For this review, take the finished solid that the model builds, in its own axes (mm). A direction names the side the tool comes from. Coordinates: 2 decimals unless noted, no trailing zeros. Write each loop counter-clockwise with the first axis right and the second up, starting at its lowest first coordinate (ties: lowest second). Pieces come first, ordered by that corner, then holes. Notation, with made-up numbers: (-30, 89.25) -> (10, 89.25) arc R24 cw to (10, 124.25) -> close; hole circle Ø6 at (50.5, 87). An arc over 180 degrees is marked (long way). One line per item, written item: value. Start each with the question number.
1) For probe 1 along Y at (x, z) = (1.15, 20); probe 2 along Z at (x, y) = (0.65, 2); probe 3 along Z at (x, y) = (-0.95, 3), list the stretches that pass through material, from the lowest coordinate up. Write a range as from..to.
2) Mouldability with a two-part tool opening along Z and no side actions: class faces 1 (the flat face through (0, -3, 7)), 2 (the cylindrical face through (1.34, 3.45, 27.23)), 3 (the cylindrical face through (1.4, -1.5, -13.1)) as released by +Z, released by -Z, zero draft, split by the parting line, or undercut.
3) Add section A-A (y = -1). State the section outline as (x, z) points, and give its area (3 significant figures).
4) For pin 1 Ø4 at (y, z) = (0, 0) entering from -X; pin 2 Ø4 at (y, z) = (0, 15) entering from -X; pin 3 Ø1.5 at (x, z) = (1, 0) entering from +Y; pin 4 Ø4 at (y, z) = (3, 20.5) entering from -X, all flat-tipped, find the tip position at first contact; note any pin that passes through.
5) Machinability: for faces 4 (the cylindrical face through (-1.4, -1.5, -13.1)), 5 (the flat face through (0, 6, -12)), 6 (the cylindrical face through (-0.38, 2.96, -13.59)), which of the approach directions +Z, -Z, +X, -X, +Y, -Y give a long, thin tool a straight path to every point of the face, cutting with its end or side? Answer none if there is none.
6) Add section C-C (y = 1). State the section outline as (x, z) points.
7) Add section D-D (z = 11.5). State the section outline as (x, y) points.
Solid Edge part; units mm, degrees
sketch "Sketch1" plane through (0, 0, 0) normal (0, -1, 0) x (1, 0, 0)
  line L0 (-1.9529, -13.631) -> (-2.5525, 27.619)
  line L1 (0, 27.619) -> (-2.5525, 27.619)
  line L2 (0, 27.619) -> (2.5525, 27.619)
  line L3 (2.5525, 27.619) -> (1.9529, -13.631)
  line L4 (0, -13.631) -> (1.9529, -13.631)
  line L5 (0, -13.631) -> (-1.9529, -13.631)
extrude "ExtrudedProtrusion_1" add sketch "Sketch1" along normal blind 3
sketch "Sketch2" plane through (0, 0, 0) normal (0, -1, 0) x (1, 0, 0)
  circle A0 centre (0, 25.119) radius 2.5
extrude "Protusion_2" add sketch "Sketch2" against normal blind 7
sketch "Sketch3" plane through (0, 0, 0) normal (0, -1, 0) x (1, 0, 0)
  circle A0 centre (0, -11.881) radius 1.75
extrude "ExtrudedProtrusion_3" add sketch "Sketch3" against normal blind 6
fillet "Round1" radius 2.3 2 edges at (2.5525, -1.5, 27.619) (-2.5525, -1.5, 27.619)
fillet "Round_2" radius 1.9 2 edges at (1.9529, -1.5, -13.631) (-1.9529, -1.5, -13.631)
Numbers:
1. probe 1: -3..0
1. probe 2: -13.51..-10.26, 22.7..27.53
1. probe 3: -13.35..-10.41, 22.81..27.43
2. face 1: zero draft
2. face 2: undercut
2. face 3: released by -Z
3. outline: (-2.52, 25.29) -> (-1.98, -11.76) arc R1.9 ccw to (-0.08, -13.63) -> (0.08, -13.63) arc R1.9 ccw to (1.98, -11.76) -> (2.52, 25.29) arc R2.3 ccw to (0.22, 27.62) -> (-0.22, 27.62) arc R2.3 ccw to start
3. area: 182 mm²
4. pin 1: x = -2.18
4. pin 2: x = -2.4
4. pin 3: y = 0
4. pin 4: through
5. face 4: -Z, -X, +Y, -Y
5. face 5: -Z, +X, -X, +Y
5. face 6: +Y
6. outline: circle Ø5 at (0, 25.12); circle Ø3.5 at (0, -11.88)
7. outline: (-2.32, -3) -> (2.32, -3) -> (2.32, 0) -> (-2.32, 0) -> close
